The listing builds one solid part. Answer for the finished solid, in the listing's coordinates (mm). A direction names the side the tool comes from. Coordinates: 2 decimals unless noted, no trailing zeros. Order: outer loops, then holes, each group sorted by start corner. A loop starts at its lowest first (then second) coordinate and runs counter-clockwise, first axis right, second up. Notation, with made-up numbers: (63, -21) -> (115, -21) arc R11 cw to (115, -13) -> close; hole circle Ø8 at (25, 45). An arc over 180 degrees is marked (long way). Answer in a Markdown table with one row per item. Add a question column.
```python
from build123d import *

# Parameters (mm, degrees)
CHAMFER1_SIZE = 0.127


with BuildPart() as part:
    # Sketch1 → Revolve1 (revolve)
    with BuildSketch(Plane.XY, mode=Mode.PRIVATE) as revolve1_sk:
        Polygon((6.3627, 0), (19.446875, 0), (19.446875, 1.5875), (15.24, 1.5875), (15.24, 28.575), (19.446875, 28.575), (19.446875, 30.1625), (6.3627, 30.1625), (6.3627, 25.3873), (5.08, 25.3873), (5.08, 4.7752), (6.3627, 4.7752), align=None)
    revolve(revolve1_sk.sketch.rotate(Axis((0, 30.1625, 0), (0, -1, 0)), 90), axis=Axis((0, 30.1625, 0), (0, -1, 0)))

    # Chamfer1
    chamfer1_edges = [part.edges().sort_by_distance(p)[0] for p in [
        (0, 4.7752, -5.08),
        (0, 25.3873, -5.08),
        (0, 30.1625, -6.3627),
        (0, 30.1625, -19.446875),
        (0, 28.575, -19.446875),
        (0, 1.5875, -19.446875),
        (0, 0, -19.446875),
        (0, 0, -6.3627),
    ]]
    chamfer(chamfer1_edges, length=CHAMFER1_SIZE)


solid = part.part
```
Q1. Straight lines are drawn through the part: line 1 (X direction, y = 3.7, z = 0); line 2 (X direction, y = 15.5, z = 0); line 3 (Y direction, x = -9.5, z = -14) (1 decimal). For each, find the intervals that lie inside material, in ascending order.
Q2. Determine the mould class of faces 1 (the face through (-15.11, 15.27, -1.98)), 2 (the face through (8, 30.162, 0)), 3 (the face through (5, 25.387, -2)) for opening direction X: +X half, -X half, draft (parallel to the pull), parting line (faces both ways), or undercut.
Q3. A cutting plane is placed at B-B (y = 15). Determine the outline of the cut face in (x, z).
Q4. Given pin 1 (2 mm diameter, centred on x = -4.5, y = 26, fed in from -Z); pin 2 (1 mm diameter, centred on x = -0.5, y = 24, fed in from +Z); pin 3 (5 mm diameter, centred on y = 21.5, z = -12, fed in from +X), each flat-ended and moving along its own axis, determine where each tip first touches the part or whether it passes through.
Q5. A cutting plane is placed at A-A (y = 3.5). Determine the outline of the cut face in (x, z).
Q6. For faces 4 (the face through (5.6, 1.587, -14.4)), 5 (the face through (-6.31, 27.68, -0.83)), 6 (the face through (-6.31, 2.42, -0.83)), determine the directions among +Z, -Z, +X, -X, +Y, -Y from which every point of the face is accessible in a straight line to the end or side of a thin tool.
Returned:
| question | item | result |
|---|---|---|
| 1 | line 1 | x = -15.24 to -6.36, 6.36 to 15.24 |
| 1 | line 2 | x = -15.24 to -5.08, 5.08 to 15.24 |
| 1 | line 3 | y = 0 to 1.6, 28.6 to 30.2 |
| 2 | face 1 | parting line |
| 2 | face 2 | draft |
| 2 | face 3 | undercut |
| 3 | outline | circle Ø30.48 at (0, 0); hole circle Ø10.16 at (0, 0) |
| 4 | pin 1 | stops at z = -14.83 |
| 4 | pin 2 | stops at z = 15.24 |
| 4 | pin 3 | stops at x = 11.92 |
| 5 | outline | circle Ø30.48 at (0, 0); hole circle Ø12.73 at (0, 0) |
| 6 | face 4 | none |
| 6 | face 5 | +Y |
| 6 | face 6 | -Y |
